from build123d import *

# Parameters (mm, degrees)
F1_DEPTH = 6
F0_W     = 51.6
F0_H     = 15
F2_DEPTH = 1


with BuildPart() as f1:
    # F0 (on Top) → F1 (new body)
    with BuildSketch(Plane.XY):
        with BuildLine():
            Line((30.75, -5), (30.75, 10))
            Line((30.75, 10), (25.8, 10))
            Line((25.8, 10), (25.8, -5))
            Line((25.8, -5), (-25.8, -5))
            Line((-25.8, -5), (-25.8, 10))
            Line((-25.8, 10), (-30.75, 10))
            Line((-30.75, 10), (-30.75, -5))
            ThreePointArc((-30.75, -5), (-29.285534, -8.535534), (-25.75, -10))
            Line((-25.75, -10), (25.75, -10))
            ThreePointArc((25.75, -10), (29.285534, -8.535534), (30.75, -5))
        make_face()
    extrude(amount=F1_DEPTH)

    # F0 (on Top) → F2 (join)
    with BuildSketch(Plane.XY):
        with Locations((0, 2.5)):
            Rectangle(F0_W, F0_H)
        with BuildLine():
            Line((30.75, -5), (30.75, 10))
            Line((30.75, 10), (25.8, 10))
            Line((25.8, 10), (25.8, -5))
            Line((25.8, -5), (-25.8, -5))
            Line((-25.8, -5), (-25.8, 10))
            Line((-25.8, 10), (-30.75, 10))
            Line((-30.75, 10), (-30.75, -5))
            ThreePointArc((-30.75, -5), (-29.285534, -8.535534), (-25.75, -10))
            Line((-25.75, -10), (25.75, -10))
            ThreePointArc((25.75, -10), (29.285534, -8.535534), (30.75, -5))
        make_face()
    extrude(amount=-F2_DEPTH)


solid = f1.part
Geometry check sheet. Reference: the model listing, model coordinates, mm. A direction names the side the tool comes from. Give positions to 0.01 mm unless a question says otherwise; leave off trailing zeros. Order: outer loops, then holes, each group sorted by start corner. A loop starts at its lowest first (then second) coordinate and runs counter-clockwise, first axis right, second up.
1) Cross-section at A-A (x = 20.5). Record the boundary of the cut face in (y, z), then the cut area to 3 significant figures.
Results are:
outline: (-10, -1) - (10, -1) - (10, 0) - (-5, 0) - (-5, 6) - (-10, 6) - close
area: 50.0 mm2
2) Gauge pin test, flat ends, axial feed: pin 1 (1.5 mm diameter, centred on y = -7.5, z = 4.5, fed in from +X); pin 2 (7.5 mm diameter, centred on x = -4, y = 2, fed in from +Z). Record the tip position at first contact, or that the pin passes through.
Results are:
pin 1: stops at x = 30.43
pin 2: stops at z = 0
3) Tool access check on faces 4 (the flat face through (-30.75, 3, 3)), 5 (the flat face through (0, -5, 3)). Record the directions out of +Z, -Z, +X, -X, +Y, -Y that give a thin tool (end or side, any length) a straight path to the whole face; none if there is none.
Results are:
face 4: +Z, -Z, -X, +Y, -Y
face 5: +Z, +Y
4) Cross-section at C-C (y = -0.25). Record the boundary of the cut face in (x, z).
Results are:
outline: (-30.75, -1) - (30.75, -1) - (30.75, 6) - (25.8, 6) - (25.8, 0) - (-25.8, 0) - (-25.8, 6) - (-30.75, 6) - close
5) Cross-section at B-B (z = 1.75). Record the boundary of the cut face in (x, y), then the cut area to 3 significant figures.
Results are:
outline: (-30.75, -5) arc R5 ccw to (-25.75, -10) - (25.75, -10) arc R5 ccw to (30.75, -5) - (30.75, 10) - (25.8, 10) - (25.8, -5) - (-25.8, -5) - (-25.8, 10) - (-30.75, 10) - close
area: 445 mm2
6) Draft check along X on faces 1 (the flat face through (0, 3, 0)), 2 (the flat face through (0, -10, 3)), 3 (the cylindrical face through (29.25, -8.57, 2.55)). Enter one of: released by +X, released by -X, zero draft, split by the parting line, or undercut.
Results are:
face 1: undercut
face 2: zero draft
face 3: released by +X
7) Material ranges on probe 1 along X at (y, z) = (0, 5); probe 2 along Z at (x, y) = (20, 1.5); probe 3 along Y at (x, z) = (14.5, 3.5), recorded low to high.
Results are:
probe 1: x = -30.75 to -25.8, 25.8 to 30.75
probe 2: z = -1 to 0
probe 3: y = -10 to -5
